from build123d import *

# Parameters (mm, degrees)
SKETCH1_R               = 5.5
BOSS_EXTRUDE1_DEPTH     = 2
BOSS_EXTRUDE1_2_DEPTH   = 2
BOSS_EXTRUDE1_3_DEPTH   = 2
BOSS_EXTRUDE1_4_DEPTH   = 2
BOSS_EXTRUDE1_5_DEPTH   = 2
BOSS_EXTRUDE1_6_DEPTH   = 2
BOSS_EXTRUDE2_START     = -5
BOSS_EXTRUDE2_OUTLINE_R = 1.7
BOSS_EXTRUDE2_DEPTH     = 5
CUT_EXTRUDE1_DEPTH      = 1


# Read off the part's stored shape, not the designer's step: Boss-Extrude2
with BuildPart() as part:
    # Sketch1 → Boss-Extrude1 (new body)
    with BuildSketch(Plane(origin=(0, 0, 0), x_dir=(1, 0, 0), z_dir=(0, 1, 0))):
        Polygon((3.686387934, -16.664883738), (3.686388262, -4.664883738), (-8.313611738, -4.66488341), (-8.313612066, -16.66488341), align=None)
        with Locations(Location((-2.313611902, -10.664883574, 0), (0, 0, 270))):
            Circle(SKETCH1_R, mode=Mode.SUBTRACT)
    extrude(amount=-BOSS_EXTRUDE1_DEPTH)



with BuildPart() as body_2:
    # Sketch1 → Boss-Extrude1 2 (new body)
    with BuildSketch(Plane(origin=(0, 0, 0), x_dir=(1, 0, 0), z_dir=(0, 1, 0))):
        Polygon((19.086387939, -16.664884095), (19.086388267, -4.664884095), (7.086388267, -4.664883767), (7.086387939, -16.664883767), align=None)
        with Locations(Location((13.086388103, -10.664883931, 0), (0, 0, 270))):
            Circle(SKETCH1_R, mode=Mode.SUBTRACT)
    extrude(amount=-BOSS_EXTRUDE1_2_DEPTH)


with BuildPart() as body_3:
    # Sketch1 → Boss-Extrude1 3 (new body)
    with BuildSketch(Plane(origin=(0, 0, 0), x_dir=(1, 0, 0), z_dir=(0, 1, 0))):
        Polygon((34.486387949, -16.66488445), (34.486388277, -4.66488445), (22.486388277, -4.664884122), (22.486387949, -16.664884122), align=None)
        with Locations(Location((28.486388113, -10.664884286, 0), (0, 0, 270))):
            Circle(SKETCH1_R, mode=Mode.SUBTRACT)
    extrude(amount=-BOSS_EXTRUDE1_3_DEPTH)


with BuildPart() as body_4:
    # Sketch1 → Boss-Extrude1 4 (new body)
    with BuildSketch(Plane(origin=(0, 0, 0), x_dir=(1, 0, 0), z_dir=(0, 1, 0))):
        Polygon((14.786387887, -17.664883977), (14.786387559, -29.664883977), (26.786387559, -29.664884305), (26.786387887, -17.664884305), align=None)
        with Locations(Location((20.786387723, -23.664884141, 0), (0, 0, 270))):
            Circle(SKETCH1_R, mode=Mode.SUBTRACT)
    extrude(amount=-BOSS_EXTRUDE1_4_DEPTH)


with BuildPart() as body_5:
    # Sketch1 → Boss-Extrude1 5 (new body)
    with BuildSketch(Plane(origin=(0, 0, 0), x_dir=(1, 0, 0), z_dir=(0, 1, 0))):
        Polygon((30.186386338, -17.664884333), (30.18638601, -29.664884333), (42.18638601, -29.664884661), (42.186386338, -17.664884661), align=None)
        with Locations(Location((36.186386174, -23.664884497, 0), (0, 0, 270))):
            Circle(SKETCH1_R, mode=Mode.SUBTRACT)
    extrude(amount=-BOSS_EXTRUDE1_5_DEPTH)


with BuildPart() as body_6:
    # Sketch1 → Boss-Extrude1 6 (new body)
    with BuildSketch(Plane(origin=(0, 0, 0), x_dir=(1, 0, 0), z_dir=(0, 1, 0))):
        Polygon((-0.613612103, -17.664883618), (-0.613612431, -29.664883618), (11.386387569, -29.664883947), (11.386387897, -17.664883947), align=None)
        with Locations(Location((5.386387733, -23.664883782, 0), (0, 0, 270))):
            Circle(SKETCH1_R, mode=Mode.SUBTRACT)
    extrude(amount=-BOSS_EXTRUDE1_6_DEPTH)


with BuildPart() as part_1:
    add(part.part)

    add(body_2.part)  # Boss-Extrude2 merges body 2

    add(body_3.part)  # Boss-Extrude2 merges body 3

    add(body_4.part)  # Boss-Extrude2 merges body 4

    add(body_5.part)  # Boss-Extrude2 merges body 5

    add(body_6.part)  # Boss-Extrude2 merges body 6
    # Boss-Extrude2 outline → Boss-Extrude2 (add)
    with BuildSketch(Plane(origin=(0, 0, 0), x_dir=(1, 0, 0), z_dir=(0, 1, 0)).offset(BOSS_EXTRUDE2_START)):
        Polygon((11.386387569, -29.664883947), (7.886387562, -29.664883851), (7.886387555, -30.164883851), (18.286387545, -30.164884073), (18.286387559, -29.664884073), (14.786387559, -29.664883977), (14.786387887, -17.664883977), (26.786387887, -17.664884305), (26.786387559, -29.664884305), (23.286387552, -29.66488421), (23.286387545, -30.16488421), (33.686385997, -30.164884494), (33.68638601, -29.664884428), (30.18638601, -29.664884333), (30.186386338, -17.664884333), (42.186386338, -17.664884661), (42.18638601, -29.664884661), (38.686386004, -29.664884565), (38.686385997, -30.164884565), (52.936387554, -30.164884954), (52.936388265, -4.164885084), (30.986388291, -4.164884354), (30.986388277, -4.664884354), (34.486388277, -4.66488445), (34.486387949, -16.66488445), (22.486387949, -16.664884122), (22.486388277, -4.664884122), (25.986388284, -4.664884218), (25.986388291, -4.164884218), (15.586388281, -4.164884108), (15.586388267, -4.664883999), (19.086388267, -4.664884095), (19.086387939, -16.664884095), (7.086387939, -16.664883767), (7.086388267, -4.664883767), (10.586388274, -4.664883862), (10.586388281, -4.164883862), (0.186388276, -4.164883578), (0.186388262, -4.664883642), (3.686388262, -4.664883738), (3.686387934, -16.664883738), (-8.313612066, -16.66488341), (-8.313611738, -4.66488341), (-4.813611731, -4.664883505), (-4.813611724, -4.164883505), (-19.063611735, -4.164883116), (-19.063612446, -30.164883114), (2.886387555, -30.164883714), (2.886387569, -29.664883714), (-0.613612431, -29.664883618), (-0.613612103, -17.664883618), (11.386387897, -17.664883947), align=None)
        with Locations((47.93638791, -17.164884883)):
            Circle(BOSS_EXTRUDE2_OUTLINE_R, mode=Mode.SUBTRACT)
        with Locations((-14.06361209, -17.164883252)):
            Circle(BOSS_EXTRUDE2_OUTLINE_R, mode=Mode.SUBTRACT)
    extrude(amount=BOSS_EXTRUDE2_DEPTH)

    # Sketch2 → Cut-Extrude1 (cut)
    # profile 1 of 2: a face of its own
    with BuildSketch(Plane(origin=(0, -5, 0), x_dir=(-1, 0, 0), z_dir=(0, -1, 0))):
        Polygon((6.544081332, -23.739762668), (8.090876204, -23.739762668), (8.090876204, -24.065403693), (6.829017229, -24.065403693), (6.829017229, -25.04232677), (8.090876204, -25.04232677), (8.090876204, -25.367967796), (6.829017229, -25.367967796), (6.829017229, -26.914762668), (6.544081332, -26.914762668), align=None)
    # profile 2 of 2: a face of its own
    with BuildSketch(Plane(origin=(0, -5, 0), x_dir=(-1, 0, 0), z_dir=(0, -1, 0))):
        Polygon((10.108960138, -23.658352411), (10.166837742, -23.658352411), (10.166837742, -25.856429335), (10.533183896, -25.856429335), (10.533183896, -26.18207036), (10.166837742, -26.18207036), (10.166837742, -26.914762668), (9.881901845, -26.914762668), (9.881901845, -26.18207036), (8.375812101, -26.18207036), align=None)
        Polygon((9.881901845, -25.856429335), (9.881901845, -24.478815152), (8.936143631, -25.856429335), align=None, mode=Mode.SUBTRACT)
    extrude(amount=-CUT_EXTRUDE1_DEPTH, mode=Mode.SUBTRACT)


solid = part_1.part
Geometry check sheet. Reference: the model listing, model coordinates, mm. A direction names the side the tool comes from. Give positions to 0.01 mm unless a question says otherwise; leave off trailing zeros. Order: outer loops, then holes, each group sorted by start corner. A loop starts at its lowest first (then second) coordinate and runs counter-clockwise, first axis right, second up.
1. Sectioned sample at B-B (x = -13). Record the boundary of the cut face in (y, z).
Completed:
outline: (-5, 4.16) - (0, 4.16) - (0, 15.84) - (-5, 15.84) - close; (-5, 18.49) - (0, 18.49) - (0, 30.16) - (-5, 30.16) - close
2. Sectioned sample at C-C (x = 16.5). Record the boundary of the cut face in (y, z), then the cut area to 3 significant figures.
Completed:
outline: (-5, 4.16) - (0, 4.16) - (0, 6.35) - (-2, 6.35) - (-2, 4.66) - (-5, 4.66) - close; (-5, 16.66) - (-2, 16.66) - (-2, 14.98) - (0, 14.98) - (0, 20.22) - (-2, 20.22) - (-2, 17.66) - (-5, 17.66) - close; (-5, 29.66) - (-2, 29.66) - (-2, 27.11) - (0, 27.11) - (0, 30.16) - (-5, 30.16) - close
area: 27.0 mm2
3. Draft check along Y on faces 4 (the face through (26, -2, 16)), 5 (the face through (29, -1, 4.665)). Enter one of: pulls with the +Y half, pulls with the -Y half, needs draft (parallel to the pull), parting line crosses it, or undercut.
Completed:
face 4: pulls with the -Y half
face 5: needs draft
4. Sectioned sample at A-A (z = 21.75). Record the boundary of the cut face in (x, y).
Completed:
outline: (-19.06, -5) - (-0.61, -5) - (-0.61, -2) - (0.23, -2) - (0.23, 0) - (-19.06, 0) - close; (10.54, -2) - (11.39, -2) - (11.39, -5) - (14.79, -5) - (14.79, -2) - (15.63, -2) - (15.63, 0) - (10.54, 0) - close; (25.94, -2) - (26.79, -2) - (26.79, -5) - (30.19, -5) - (30.19, -2) - (31.03, -2) - (31.03, 0) - (25.94, 0) - close; (41.34, -2) - (42.19, -2) - (42.19, -5) - (52.94, -5) - (52.94, 0) - (41.34, 0) - close
5. Access from +Z, -Z, +X, -X, +Y, -Y to the whole of each face (thin tool, end or side, straight path). Record for faces 1 (the face through (-19.064, -3, 17)), 2 (the face through (21, -1, 29.665)), 3 (the face through (36, -4, 17.665)).
Completed:
face 1: +Z, -Z, -X, +Y, -Y
face 2: +Z, +Y, -Y
face 3: -Y
6. Scan lines: line 1 (X direction, y = -2.55, z = 19.25); line 2 (Z direction, x = 25, y = -4.3); line 3 (X direction, y = -3.1, z = 10.75). Record each from-to range of solid material in increasing order.
Completed:
line 1: x = -19.06 to -0.61, 11.39 to 14.79, 26.79 to 30.19, 42.19 to 52.94
line 2: z = 4.16 to 4.66, 16.66 to 17.66, 29.66 to 30.16
line 3: x = -19.06 to -8.31, 3.69 to 7.09, 19.09 to 22.49, 34.49 to 52.94
7. Depth check by flat-ended pin: pin 1 (2 mm diameter, centred on x = 5, y = -1.5, fed in from +Z). Enter the tip coordinate at first touch or a pass-through.
Completed:
pin 1: stops at z = 29.66
8. Sectioned sample at D-D (y = -1). State how many separate pieces and enclosed holes the cut face has, then the cut area to 3 significant figures.
Completed:
separate pieces: 1
enclosed holes: 8
area: 1,270 mm2
